Study the drawing (mm; zero at the part's minimum x, y, z) and answer. A direction names the side the tool comes from. Coordinates: 2 decimals unless noted, no trailing zeros. Order: outer loops, then holes, each group sorted by start corner. A loop starts at its lowest first (then second) coordinate and runs counter-clockwise, first axis right, second up. Notation, with made-up numbers: M 1.25,4 L 21.25,4 A25 ccw 21.25,31 Z; hole C 0.5,32 d2. An arc over 180 degrees is marked long. Use a Markdown table: item, result. Add a question column.
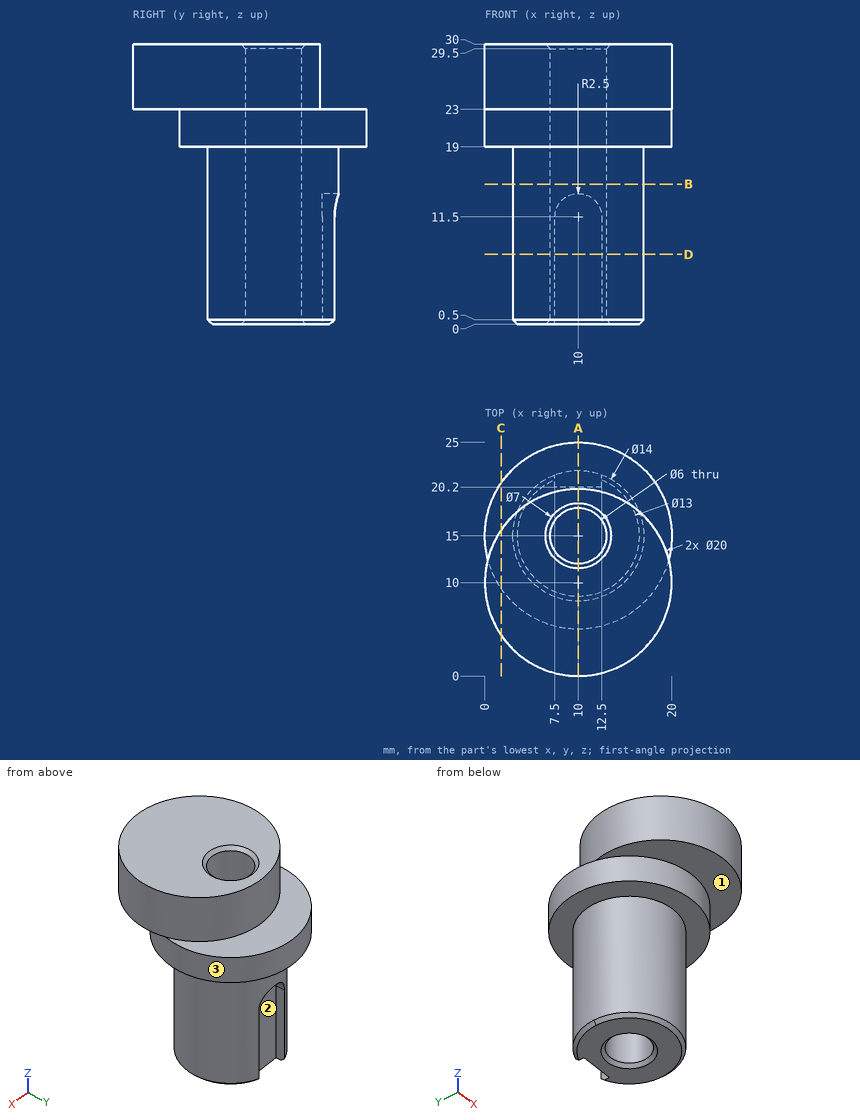
(1) Straight lines are drawn through the part: line 1 (Y direction, x = 10, z = 7.75); line 2 (Y direction, x = 10, z = 23.5); line 3 (Z direction, x = 14.25, y = 8.75). For each, find the intervals that lie inside material, in ascending order.
(2) Which of the six approach directions +Z, -Z, +X, -X, +Y, -Y give full straight-line access (tool end or side, diameter ignored) to the marked faces 1, 2 and 3?
(3) A cutting plane is placed at C-C on x = 1.75. Write down the section's boundary in (y, z).
(4) A cutting plane is placed at A-A on x = 10. Write down the section's boundary in (y, z).
(5) A cutting plane is placed at D-D on z = 7.5. Write down the section's boundary in (x, y).
(6) A cutting plane is placed at B-B on z = 15. Write down the section's boundary in (x, y), plus the area to 3 significant figures.
(7) Given P1, Ø4, axis at x = 10, z = 6.5, coming from the +Y side; P2, Ø8, axis at y = 8.5, z = 12, coming from the -X side; P3, Ø1.1, axis at y = 21, z = 5.5, coming from the +X side; P4, Ø5.5, axis at x = 10, y = 15, coming from the +Z side, each flat-ended and moving along its own axis, determine where each tip first touches the part or whether it passes through.
From the geometry:
| question | item | result |
|---|---|---|
| 1 | line 1 | y = 8 to 12, 18 to 20.2 |
| 1 | line 2 | y = 0 to 12, 18 to 20 |
| 1 | line 3 | z = 19 to 30 |
| 2 | face 1 | -Z, -Y |
| 2 | face 2 | -Z, +Y |
| 2 | face 3 | -Z |
| 3 | outline | M 4.35,23 L 9.35,23 L 9.35,19 L 20.65,19 L 20.65,23 L 15.65,23 L 15.65,30 L 4.35,30 Z |
| 4 | outline | M 0,23 L 5,23 L 5,19 L 8,19 L 8,0.5 L 8.5,0 L 11.5,0 L 12,0.5 L 12,29.5 L 11.5,30 L 0,30 Z; M 18,0.5 L 18.5,0 L 20.2,0 L 20.2,14 L 22,14 L 22,19 L 25,19 L 25,23 L 20,23 L 20,30 L 18.5,30 L 18,29.5 Z |
| 5 | outline | M 7.5,20.2 L 7.5,21.54 A7 ccw long 12.5,21.54 L 12.5,20.2 Z; hole C 10,15 d6 |
| 6 | outline | C 10,15 d14; hole C 10,15 d6 |
| 6 | area | 126 mm2 |
| 7 | P1 | stops at y = 20.2 |
| 7 | P2 | stops at x = 3.46 |
| 7 | P3 | stops at x = 14.39 |
| 7 | P4 | passes through |
